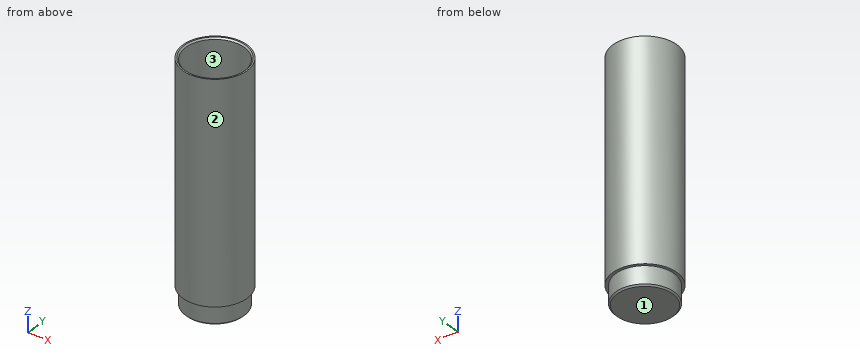
from build123d import *

# Parameters (mm, degrees)
F1_R     = 17
F1_R_2   = 15.5
F2_DEPTH = 115
F3_SIZE  = 0.75
F4_R     = 17
F5_DEPTH = 2
F6_R     = 15.5
F7_DEPTH = 10
F8_SIZE  = 0.75


with BuildPart() as f2:
    # F1 (on offset) → F2 (new body)
    with BuildSketch(Plane.XY.offset(222)):
        Circle(F1_R)
        Circle(F1_R_2, mode=Mode.SUBTRACT)
    extrude(amount=F2_DEPTH)

    # F3
    f3_edges = [f2.edges().sort_by_distance(p)[0] for p in [
        (-15.5, 0, 337),
    ]]
    chamfer(f3_edges, length=F3_SIZE)

    # F4 (on offset) → F5 (join)
    with BuildSketch(Plane.XY.offset(222)):
        Circle(F4_R)
    extrude(amount=F5_DEPTH)

    # F6 (on face) → F7 (join)
    with BuildSketch(Plane(origin=(0, 0, 222), x_dir=(1, 0, 0), z_dir=(0, 0, -1))):
        Circle(F6_R)
    extrude(amount=F7_DEPTH)

    # F8
    f8_edges = [f2.edges().sort_by_distance(p)[0] for p in [
        (-15.5, 0, 212),
    ]]
    chamfer(f8_edges, length=F8_SIZE)


solid = f2.part
The model under review builds one solid part; all positions refer to its coordinate system, in mm. Face numbers are marked on the shaded views. Coordinates: 2 decimals unless noted, no trailing zeros. Loops run counter-clockwise (first coordinate to the right, second up) from the corner with the lowest first, then second, coordinate; pieces in that order, holes last.
(1) Insertion check: P1, Ø4, axis at x = -10.5, z = 316.5, coming from the -Y side; P2, Ø10, axis at y = -7.5, z = 234, coming from the +X side; P3, Ø8, axis at y = -13, z = 323.5, coming from the +X side. Each pin has a flat end and moves straight along its axis. Give the tip position at first contact, or say it passes through.
Determined:
P1: stops at y = -14.72
P2: stops at x = 16.82
P3: stops at x = 14.42
(2) Wall thickness on L1, parallel to Y at x = 0, z = 250.5; L2, parallel to Z at x = -1, y = 8; L3, parallel to Y at x = 7, z = 301: over which ranges is each line inside the solid? List them lowest first.
Determined:
L1: y = -17 to -15.5, 15.5 to 17
L2: z = 212 to 224
L3: y = -15.49 to -13.83, 13.83 to 15.49
(3) Consider section A-A, the plane y = 0. Give the boundary of the cut face in (x, z), plus the area to 3 significant figures.
Determined:
outline: (-17, 222) - (-15.5, 222) - (-15.5, 212.75) - (-14.75, 212) - (14.75, 212) - (15.5, 212.75) - (15.5, 222) - (17, 222) - (17, 337) - (16.25, 337) - (15.5, 336.25) - (15.5, 224) - (-15.5, 224) - (-15.5, 336.25) - (-16.25, 337) - (-17, 337) - close
area: 716 mm2
(4) Consider section C-C, the plane z = 232. Give the boundary of the cut face in (x, y), plus the area to 3 significant figures.
Determined:
outline: circle Ø34 at (0, 0); hole circle Ø31 at (0, 0)
area: 153 mm2
(5) Draft analysis for pull direction Y (two halves, no side actions). For the marked faces 1, 2 and 3, state which applies: +Y half, -Y half, draft (parallel to the pull), parting line (faces both ways), or undercut.
Determined:
face 1: draft
face 2: parting line
face 3: undercut
